```python
from build123d import *

# Parameters (mm, degrees)
SKETCH1_W           = 8.466666667
SKETCH1_H           = 8.466666667
BOSS_EXTRUDE1_DEPTH = 8.466666667
CUT_EXTRUDE1_DEPTH  = 6.35
CHAMFER1_SIZE       = 0.635


with BuildPart() as part:
    # Sketch1 → Boss-Extrude1 (new body)
    with BuildSketch(Plane(origin=(0, 0, 0), x_dir=(1, 0, 0), z_dir=(0, 1, 0))):
        with Locations((4.233333334, 4.233333334)):
            Rectangle(SKETCH1_W, SKETCH1_H)
    extrude(amount=BOSS_EXTRUDE1_DEPTH)

    # Sketch3 → Cut-Extrude1 (cut)
    with BuildSketch(Plane.XY):
        Polygon((1.058333333, 4.233333333), (4.233333333, 1.058333333), (7.408333333, 4.233333333), (4.233333333, 7.408333333), align=None)
    extrude(amount=-CUT_EXTRUDE1_DEPTH, mode=Mode.SUBTRACT)

    # Chamfer1
    chamfer1_edges = [part.edges().sort_by_distance(p)[0] for p in [
        (2.645833333, 5.820833333, -6.35),
        (5.820833333, 5.820833333, -6.35),
        (5.820833333, 2.645833333, -6.35),
        (2.645833333, 2.645833333, -6.35),
        (2.645833333, 5.820833333, 0),
        (2.645833333, 2.645833333, 0),
        (5.820833333, 2.645833333, 0),
        (5.820833333, 5.820833333, 0),
    ]]
    chamfer(chamfer1_edges, length=CHAMFER1_SIZE)


solid = part.part
```
Input: part model. Units: mm. Frame: model coordinates. A direction names the side the tool comes from. Coordinates: 2 decimals unless noted, no trailing zeros. Loops run counter-clockwise (first coordinate to the right, second up) from the corner with the lowest first, then second, coordinate; pieces in that order, holes last. Notation, with made-up numbers: M -1,-19 L 43,-19 A14 ccw 43,-10 Z; hole C 25.5,47.5 d6. An arc over 180 degrees is marked long. One line per item, written item: value.
(1) Pull-direction query (Y, two-part tool) for faces 3 (the flat face through (4, 8.467, -4)), 4 (the flat face through (5.799, 2.624, -3.139)), 5 (the flat face through (8.467, 4, -4)); classes: +Y half, -Y half, draft (parallel to the pull), parting line (faces both ways), or undercut.
Filled in:
face 3: +Y half
face 4: undercut
face 5: draft
(2) Section A-A (z = -3.5). Output: boundary loops of the cut face in (x, y).
Filled in:
outline: M 0,0 L 8.47,0 L 8.47,8.47 L 0,8.47 Z; hole M 1.06,4.23 L 4.23,1.06 L 7.41,4.23 L 4.23,7.41 Z
(3) Section D-D (z = -6). Output: boundary loops of the cut face in (x, y).
Filled in:
outline: M 0,0 L 8.47,0 L 8.47,8.47 L 0,8.47 Z; hole M 1.46,4.23 L 4.23,1.46 L 7.01,4.23 L 4.23,7.01 Z
(4) Pin query (flat end, axial travel): pin 1 (5 mm diameter, centred on x = 3.5, y = 5.5, fed in from +Z); pin 2 (1.4 mm diameter, centred on x = 5, y = 5, fed in from +Z). Return the tip coordinate at first contact, or that it passes through.
Filled in:
pin 1: z = 0
pin 2: z = -6.18
(5) Section B-B (y = 3.5). Output: boundary loops of the cut face in (x, z) (3 decimals).
Filled in:
outline: M 0,-8.467 L 8.467,-8.467 L 8.467,0 L 7.573,0 L 6.675,-0.635 L 6.675,-5.715 L 5.777,-6.35 L 2.69,-6.35 L 1.792,-5.715 L 1.792,-0.635 L 0.894,0 L 0,0 Z
(6) Section C-C (x = 5). Output: boundary loops of the cut face in (y, z) (3 decimals), and give its area (3 significant figures).
Filled in:
outline: M 0,-8.467 L 8.467,-8.467 L 8.467,0 L 7.54,0 L 6.642,-0.635 L 6.642,-5.715 L 5.744,-6.35 L 2.723,-6.35 L 1.825,-5.715 L 1.825,-0.635 L 0.927,0 L 0,0 Z
area: 41.1 mm^2
(7) Reachability of faces 1 (the flat face through (4, 4, -8.467)), 2 (the flat face through (2.896, 5.615, -6.037)) from +Z, -Z, +X, -X, +Y, -Y: full face, straight path, thin tool, end or side. Return the list, or none.
Filled in:
face 1: -Z, +X, -X, +Y, -Y
face 2: +Z
(8) Line query: line 1 along Y through (x, z) = (6.5, -1.75) (3 decimals); line 2 along Z through (x, y) = (2.25, 4.5); line 3 along X through (y, z) = (1.5, -1.5) (3 decimals). Output: solid intervals per line, ascending. Write a range as from..to.
Filled in:
line 1: 0..3.325, 5.142..8.467
line 2: -8.47..-6.35
line 3: 0..3.792, 4.675..8.467
